Here's how the part is built. I have some questions about the finished solid (model axes, mm). A direction names the side the tool comes from. Coordinates: 2 decimals unless noted, no trailing zeros. Write each loop counter-clockwise with the first axis right and the second up, starting at its lowest first coordinate (ties: lowest second). Pieces come first, ordered by that corner, then holes. Notation, with made-up numbers: M 83,2.5 L 106,2.5 A29 ccw 106,40.5 Z; hole C 29,-11.75 d4. An arc over 180 degrees is marked long. Use one line per item in the form item = value. Start each with the question number.
1. I want a section at C-C, the plane z = -7. List the corners of the cut face in (x, y) for me, plus the area to 3 significant figures.
2. I want a section at B-B, the plane y = -1. List the corners of the cut face in (x, z) for me, plus the area to 3 significant figures.
3. I'm going to push flat-ended pins straight in: pin 1 Ø12 at (y, z) = (15, -25.5) entering from -X; pin 2 Ø8 at (x, z) = (0, -25) entering from +Y; pin 3 Ø1.5 at (x, z) = (2.5, -6) entering from +Y; pin 4 Ø1.5 at (x, z) = (-5.5, -9) entering from +Y. Where does each tip first touch, or does it pass through?
4. I want a section at D-D, the plane x = -15. List the corners of the cut face in (y, z) for me.
5. I want a section at A-A, the plane x = 0. List the corners of the cut face in (y, z) for me.
6. Please list where these lines run through material, in increasing order: line 1 along Z through (x, y) = (0, -17.55); line 2 along Z through (x, y) = (-1.5, 18); line 3 along X through (y, z) = (-1, 13.5). Write a range as [from, to].
7. Thinking about a two-plate mould opening in Y: for faces 1 (the face through (-15.43, -15.4, 0.52)), 2 (the face through (0, 20, 1)), 3 (the face through (-0.1, -16.2, -37.5)), which applies, released by +Y, released by -Y, zero draft, split by the parting line, or undercut?
8. On a 3-axis mill with a long thin cutter (end or side, diameter ignored), from which of +Z, -Z, +X, -X, +Y, -Y can I reach the whole of each face in a straight line? I mean faces 4 (the face through (0, -16, 1)), 5 (the face through (0, -20, 1)). Say none if no direction works.
from build123d import *

# Parameters (mm, degrees)
SALIENTE_EXTRUIR1_DEPTH       = 37.5
PERCEUSE_COLONNE_POUR_M1_61_D = 10


with BuildPart() as part:
    # Croquis1 → Saliente-Extruir1 (new body, symmetric)
    with BuildSketch(Plane.XY):
        with BuildLine():
            Line((-20, 0), (-20, -14))
            ThreePointArc((-20, -14), (-18.242640687, -18.242640687), (-14, -20))
            Line((-14, -20), (14, -20))
            ThreePointArc((14, -20), (18.242640687, -18.242640687), (20, -14))
            Line((20, -14), (20, 0))
            ThreePointArc((20, 0), (0, 20), (-20, 0))
        make_face()
        with BuildLine():
            Line((-16, 0), (-16, -14))
            ThreePointArc((-16, -14), (-15.414213562, -15.414213562), (-14, -16))
            Line((-14, -16), (14, -16))
            ThreePointArc((14, -16), (15.414213562, -15.414213562), (16, -14))
            Line((16, -14), (16, 0))
            ThreePointArc((16, 0), (0, 16), (-16, 0))
        make_face(mode=Mode.SUBTRACT)
    extrude(amount=SALIENTE_EXTRUIR1_DEPTH, both=True)

    # Perceuse à colonne pour M1.61 (through all)
    with Locations(Plane(origin=(0, -20, 0), x_dir=(-1, 0, 0), z_dir=(0, -1, 0))):
        with Locations((0, -25), (0, 25)):
            Hole(PERCEUSE_COLONNE_POUR_M1_61_D / 2)


solid = part.part
Answer list:
q1.outline = M -20,-14 A6 ccw -14,-20 L 14,-20 A6 ccw 20,-14 L 20,0 A20 ccw -20,0 Z; hole M -16,-14 A2 ccw -14,-16 L 14,-16 A2 ccw 16,-14 L 16,0 A16 ccw -16,0 Z
q1.area = 500 mm²
q2.outline = M -20,-37.5 L -16,-37.5 L -16,37.5 L -20,37.5 Z; M 16,-37.5 L 20,-37.5 L 20,37.5 L 16,37.5 Z
q2.area = 600 mm²
q3.pin_1 = -17.86
q3.pin_2 = through
q3.pin_3 = 19.92
q3.pin_4 = 19.43
q4.outline = M -19.92,-37.5 L -15.73,-37.5 L -15.73,37.5 L -19.92,37.5 Z; M 5.57,-37.5 L 13.23,-37.5 L 13.23,37.5 L 5.57,37.5 Z
q5.outline = M -20,-37.5 L -16,-37.5 L -16,-30 L -20,-30 Z; M -20,-20 L -16,-20 L -16,20 L -20,20 Z; M -20,30 L -16,30 L -16,37.5 L -20,37.5 Z; M 16,-37.5 L 20,-37.5 L 20,-30 L 16,-30 Z; M 16,-20 L 20,-20 L 20,20 L 16,20 Z; M 16,30 L 20,30 L 20,37.5 L 16,37.5 Z
q6.line_1 = [-37.5, -30], [-20, 20], [30, 37.5]
q6.line_2 = [-37.5, -29.77], [-20.23, 20.23], [29.77, 37.5]
q6.line_3 = [-20, -16], [16, 20]
q7.face_1 = undercut
q7.face_2 = released by +Y
q7.face_3 = zero draft
q8.face_4 = +Z, -Z
q8.face_5 = +Z, -Z, +X, -X, -Y
